Part print with two shaded views. Sizes in mm from the minimum x, y, z corner. A direction names the side the tool comes from. Round coordinates to 2 decimals unless told otherwise and drop trailing zeros. Loops run counter-clockwise (first coordinate to the right, second up) from the corner with the lowest first, then second, coordinate; pieces in that order, holes last. Notation, with made-up numbers: M 27,33 L 45,33 A24 cw 45,70 Z; hole C 58.25,13.25 d2. An arc over 180 degrees is marked long. Use a Markdown table: item, result. Add a question column.
Item 1: Saw through at C-C on y = 5. Write the cut outline in (x, z), then the cut area to 3 significant figures.
Item 2: Saw through at D-D on x = 11. Write the cut outline in (y, z).
Item 3: Tool access for the marked faces 1 and 2: list every direction of +Z, -Z, +X, -X, +Y, -Y with a clear straight run to the whole face (end or side of a thin tool).
Item 4: Two-plate mould, pull along X, no slides. Class the marked faces 3, 4, 5 and 6: +X half, -X half, draft (parallel to the pull), parting line (faces both ways), or undercut.
Item 5: Saw through at A-A on z = 55. Write the cut outline in (x, y) (3 decimals), then the cut area to 3 significant figures.
Item 6: Pin check, flat tips, straight feed: P1, Ø4, axis at x = 34, z = 9.5, coming from the -Y side; P2, Ø3, axis at x = 44.5, y = 21, coming from the +Z side. Stop position of each tip, or through.
Item 7: Wall check: L1, parallel to X at y = 12.75, z = 41.5; L2, parallel to X at y = 23.5, z = 45; L3, parallel to Y at x = 62.5, z = 60. Give the ranges that are in metal, low to high. Write a range as from..to.
Item 8: Saw through at B-B on y = 12.7. Write the cut outline in (x, z), then the cut area to 3 significant figures.
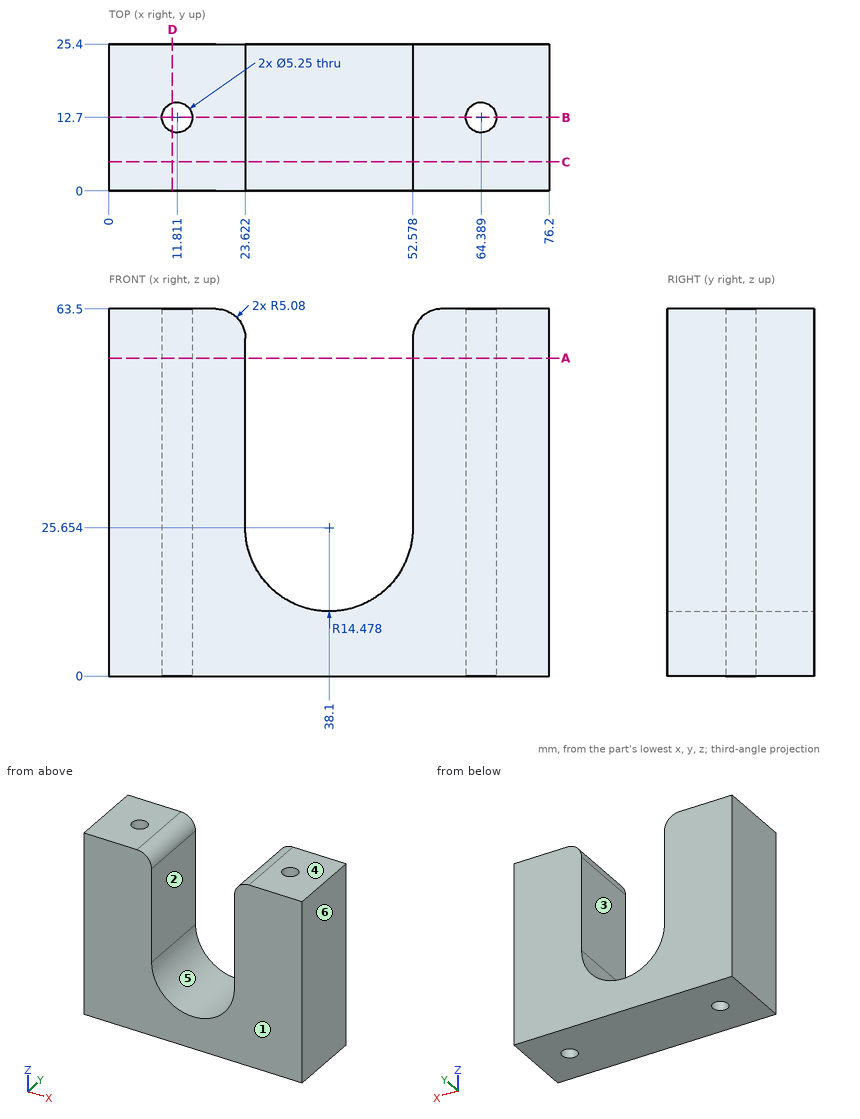
Entries:
| question | item | result |
|---|---|---|
| 1 | outline | M 0,0 L 76.2,0 L 76.2,63.5 L 57.66,63.5 A5.08 ccw 52.58,58.42 L 52.58,25.65 A14.48 cw 23.62,25.65 L 23.62,58.42 A5.08 ccw 18.54,63.5 L 0,63.5 Z |
| 1 | area | 3,400 mm2 |
| 2 | outline | M 0,0 L 10.2,0 L 10.2,63.5 L 0,63.5 Z; M 15.2,0 L 25.4,0 L 25.4,63.5 L 15.2,63.5 Z |
| 3 | face 1 | +Z, -Z, +X, -X, -Y |
| 3 | face 2 | +Z, +Y, -Y |
| 4 | face 3 | undercut |
| 4 | face 4 | draft |
| 4 | face 5 | undercut |
| 4 | face 6 | +X half |
| 5 | outline | M 0,0 L 23.622,0 L 23.622,25.4 L 0,25.4 Z; M 52.578,0 L 76.2,0 L 76.2,25.4 L 52.578,25.4 Z; hole C 11.811,12.7 d5.25; hole C 64.389,12.7 d5.25 |
| 5 | area | 1,160 mm2 |
| 6 | P1 | y = 0 |
| 6 | P2 | z = 13.52 |
| 7 | L1 | 0..9.19, 14.44..23.62, 52.58..61.76, 67.01..76.2 |
| 7 | L2 | 0..23.62, 52.58..76.2 |
| 7 | L3 | 0..10.88, 14.52..25.4 |
| 8 | outline | M 0,0 L 9.19,0 L 9.19,63.5 L 0,63.5 Z; M 14.44,0 L 61.76,0 L 61.76,63.5 L 57.66,63.5 A5.08 ccw 52.58,58.42 L 52.58,25.65 A14.48 cw 23.62,25.65 L 23.62,58.42 A5.08 ccw 18.54,63.5 L 14.44,63.5 Z; M 67.01,0 L 76.2,0 L 76.2,63.5 L 67.01,63.5 Z |
| 8 | area | 2,740 mm2 |
